For this review, take the finished solid that the model builds, in its own axes (mm). Face numbers are marked on the shaded views. Round coordinates to 2 decimals unless told otherwise and drop trailing zeros. Write each loop counter-clockwise with the first axis right and the second up, starting at its lowest first coordinate (ties: lowest second). Pieces come first, ordered by that corner, then holes. Notation, with made-up numbers: (38, -17) - (93, -17) arc R20 cw to (93, 6) - close; hole circle Ø5 at (62, 61.25). An arc over 180 degrees is marked (long way). One line per item, written item: value. Start each with the question number.
Q1. For probe 1 along X at (y, z) = (0.5, -2.5); probe 2 along X at (y, z) = (3.75, 0.5); probe 3 along X at (y, z) = (-2, 0.25), list the stretches that pass through material, from the lowest coordinate up.
Q2. Add section B-B on x = -23. Write out the cut boundary in (y, z) (1 decimal).
Q3. Add section A-A on y = -0.75. Write out the cut boundary in (x, z) (3 decimals).
Q4. Mouldability with a two-part tool opening along X and no side actions: class the marked faces 1, 2, 3 and 4 as +X half, -X half, draft (parallel to the pull), parting line (faces both ways), or undercut.
Q5. Clearance check with flat-ended pins moving along their axes: pin 1 Ø2 at (y, z) = (-2, -1) entering from +X; pin 2 Ø3.5 at (x, y) = (-22, 2.5) entering from +Z. State where each tip first meets the part, or that it passes through.
Q6. Add section C-C on y = -4. Write out the cut boundary in (x, z) (3 decimals).
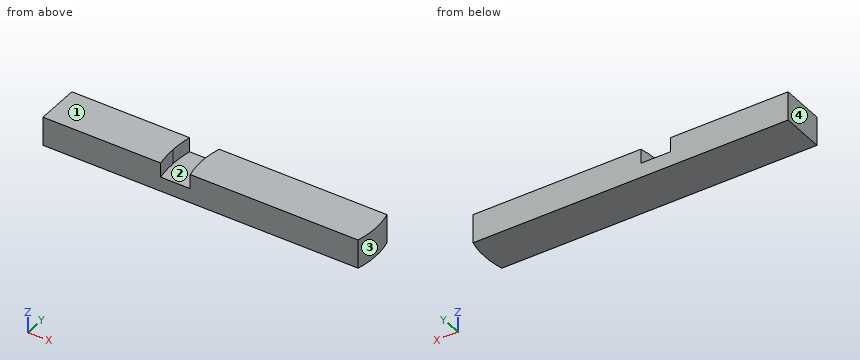
```python
from build123d import *

# Parameters (mm, degrees)
F0_W     = 36.8901663726
F0_H     = 9.525
F1_DEPTH = 3.175
F2_DEPTH = 3.175


with BuildPart() as f1:
    # F0 (on Top) → F1 (new body)
    with BuildSketch(Plane.XY):
        with BuildLine():
            ThreePointArc((18.4450831863, -4.7625), (18.8981657139, -2.4003817718), (19.05, 0))
            ThreePointArc((19.05, 0), (18.8981657139, 2.4003817718), (18.4450831863, 4.7625))
            Line((18.4450831863, 4.7625), (18.4450831863, -4.7625))
        make_face()
        Rectangle(F0_W, F0_H)
        with BuildLine():
            Line((-18.4450831863, -4.7625), (-18.4450831863, 4.7625))
            ThreePointArc((-18.4450831863, 4.7625), (-19.05, 0), (-18.4450831863, -4.7625))
        make_face()
    extrude(amount=F1_DEPTH)



with BuildPart() as f1b:
    # F0 (on Top) → F1, piece 2 (new body)
    with BuildSketch(Plane.XY):
        with BuildLine():
            ThreePointArc((-25.4, 0), (-25.2871294453, 2.3918788461), (-24.9495209122, 4.7625))
            Line((-24.9495209122, 4.7625), (-25.4, 4.7625))
            Line((-25.4, 4.7625), (-25.4, 0))
        make_face()
        with BuildLine():
            Line((-25.4, -4.7625), (-24.9495209122, -4.7625))
            ThreePointArc((-24.9495209122, -4.7625), (-25.2871294453, -2.3918788461), (-25.4, 0))
            Line((-25.4, 0), (-25.4, -4.7625))
        make_face()
        Polygon((-25.4, 0), (-25.4, 4.7625), (-50.8, 4.7625), (-50.8, -4.7625), (-25.4, -4.7625), align=None)
    extrude(amount=F1_DEPTH)


with BuildPart() as f1_1:
    add(f1.part)

    add(f1b.part)  # F2 merges F1b
    # F0 (on Top) → F2 (join)
    with BuildSketch(Plane.XY):
        with BuildLine():
            ThreePointArc((18.4450831863, -4.7625), (18.8981657139, -2.4003817718), (19.05, 0))
            ThreePointArc((19.05, 0), (18.8981657139, 2.4003817718), (18.4450831863, 4.7625))
            Line((18.4450831863, 4.7625), (18.4450831863, -4.7625))
        make_face()
        Rectangle(F0_W, F0_H)
        with BuildLine():
            Line((-18.4450831863, -4.7625), (-18.4450831863, 4.7625))
            ThreePointArc((-18.4450831863, 4.7625), (-19.05, 0), (-18.4450831863, -4.7625))
        make_face()
        with BuildLine():
            ThreePointArc((-18.4450831863, -4.7625), (-19.05, 0), (-18.4450831863, 4.7625))
            Line((-18.4450831863, 4.7625), (-24.9495209122, 4.7625))
            ThreePointArc((-24.9495209122, 4.7625), (-25.2871294453, 2.3918788461), (-25.4, 0))
            ThreePointArc((-25.4, 0), (-25.2871294453, -2.3918788461), (-24.9495209122, -4.7625))
            Line((-24.9495209122, -4.7625), (-18.4450831863, -4.7625))
        make_face()
        with BuildLine():
            ThreePointArc((-25.4, 0), (-25.2871294453, 2.3918788461), (-24.9495209122, 4.7625))
            Line((-24.9495209122, 4.7625), (-25.4, 4.7625))
            Line((-25.4, 4.7625), (-25.4, 0))
        make_face()
        with BuildLine():
            Line((-25.4, -4.7625), (-24.9495209122, -4.7625))
            ThreePointArc((-24.9495209122, -4.7625), (-25.2871294453, -2.3918788461), (-25.4, 0))
            Line((-25.4, 0), (-25.4, -4.7625))
        make_face()
        Polygon((-25.4, 0), (-25.4, 4.7625), (-50.8, 4.7625), (-50.8, -4.7625), (-25.4, -4.7625), align=None)
    extrude(amount=-F2_DEPTH)


solid = f1_1.part
```
Result set:
1. probe 1: x = -50.8 to 19.04
1. probe 2: x = -50.8 to -25.12, -18.68 to 18.68
1. probe 3: x = -50.8 to -25.32, -18.94 to 18.94
2. outline: (-4.8, -3.2) - (4.8, -3.2) - (4.8, 0) - (-4.8, 0) - close
3. outline: (-50.8, -3.175) - (19.035, -3.175) - (19.035, 3.175) - (-19.035, 3.175) - (-19.035, 0) - (-25.389, 0) - (-25.389, 3.175) - (-50.8, 3.175) - close
4. face 1: draft
4. face 2: undercut
4. face 3: +X half
4. face 4: -X half
5. pin 1: stops at x = 19.02
5. pin 2: stops at z = 0
6. outline: (-50.8, -3.175) - (18.625, -3.175) - (18.625, 3.175) - (-18.625, 3.175) - (-18.625, 0) - (-25.083, 0) - (-25.083, 3.175) - (-50.8, 3.175) - close
